Autodesk Inventor part; units mm, degrees
ref_plane "Work Plane1" through (-5, -10, -100) normal (0, 0, -1) x (0, 1, 0)
ref_plane "YZ Plane" through (0, 0, 0) normal (1, 0, 0) x (0, 1, 0)
ref_plane "XZ Plane" through (0, 0, 0) normal (0, 1, 0) x (-1, 0, 0)
sketch "Sketch1" plane through (0, 0, 0) normal (0, 0, 1) x (1, 0, 0)
  line L0 (-5, 10) -> (-5, -10)
  line L1 (-5, -10) -> (5, -10)
  line L2 (5, -10) -> (5, -4)
  line L3 (5, -4) -> (-1, -6.1838)
  line L4 (-1, -6.1838) -> (-1, 6.1838)
  line L5 (-1, 6.1838) -> (5, 4)
  line L6 (5, 4) -> (5, 10)
  line L7 (5, 10) -> (-5, 10)
  line L8 (-1, -10) -> (9, -10)
  line L9 (9, -10) -> (9, 10)
  line L10 (9, 10) -> (-1, 10)
  line L11 (-1, 10) -> (-1, -10)
  point P0 (0, 0)
  dimension "d0" = 10
ref_plane "Work Plane1" through (-5, -10, -100) normal (0, 0, -1) x (0, 1, 0)
extrude "Extrusion1" add sketch "Sketch1" against normal up to surface (100 mm away) contours L10 L9 L8 L2 L3 L4 L5 L6
sketch "Sketch2" plane through (0, 0, 0) normal (0, 0, 1) x (1, 0, 0)
  line L0 (9, 10) -> (5, 10)
  line L1 (5, 10) -> (5, 4)
  line L2 (5, 4) -> (-1, 6.1838)
  line L3 (-1, 6.1838) -> (-1, -6.1838)
  line L4 (-1, -6.1838) -> (5, -4)
  line L5 (5, -4) -> (5, -10)
  line L6 (5, -10) -> (9, -10)
  line L7 (9, -10) -> (9, 10)
  line L8 (5, -10) -> (9, -10)
  line L9 (9, -10) -> (-5, -10)
  line L10 (-5, -10) -> (-5, 10)
  line L11 (-5, 10) -> (9, 10)
  line L12 (9, 10) -> (9, -10)
  point P0 (0, 0)
  dimension "d3" = 14
  dimension "d4" = 20
extrude "Extrusion2" add sketch "Sketch2" along normal blind 3
sketch "Sketch3" plane through (9, -10, -100) normal (1, 0, 0) x (0, 0, -1)
  line L0 (-100, 16.1838) -> (-100, 3.8162)
  circle A0 centre (-94, 10) radius 1.5
  line L1 (0, 0) -> (-103, 0)
  circle A1 centre (-86, 10) radius 1.5
  circle A2 centre (-78, 10) radius 1.5
  circle A3 centre (-70, 10) radius 1.5
  circle A4 centre (-62, 10) radius 1.5
  circle A5 centre (-54, 10) radius 1.5
  circle A6 centre (-46, 10) radius 1.5
  circle A7 centre (-38, 10) radius 1.5
  circle A8 centre (-30, 10) radius 1.5
  circle A9 centre (-22, 10) radius 1.5
  circle A10 centre (-14, 10) radius 1.5
  circle A11 centre (-6, 10) radius 1.5
  point P0 (-100, 10)
  dimension "d7" = 3
  dimension "d8" = 6
  dimension "d11" = 8
extrude "Extrusion3" cut sketch "Sketch3" against normal through all
sketch "Sketch4" plane through (0, 0, 3) normal (0, 0, 1) x (1, 0, 0)
  line L0 (-5, 10) -> (-5, -10)
  line L1 (-5, 10) -> (9, -10)
  line L2 (9, 10) -> (5, 10)
  line L3 (9, -10) -> (9, 10)
  line L4 (-5, -10) -> (5, -10)
  line L5 (9, 10) -> (-5, -10)
  line L6 (-0.75, -2.75) -> (4.75, -2.75)
  line L7 (4.75, -2.75) -> (4.75, 2.75)
  line L8 (4.75, 2.75) -> (-0.75, 2.75)
  line L9 (-0.75, 2.75) -> (-0.75, -2.75)
  line L10 (-0.75, -2.75) -> (4.75, 2.75) construction
  line L11 (4.75, -2.75) -> (-0.75, 2.75) construction
  point P0 (0, 0)
  point P1 (2, 0)
  dimension "d18" = 5.5
  dimension "d19" = 5.5
extrude "Extrusion4" add sketch "Sketch4" along normal blind 7 contours L8 L5 L1 | L1 L5 L6 L9 L8 | L5 L1 L6 | L5 L8 L7 L6 L1
properties part number "prismatic link outer"
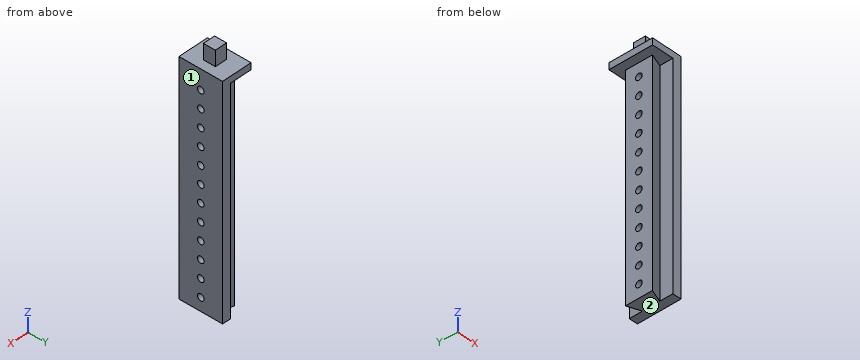
For this review, take the finished solid that the model builds, in its own axes (mm). Face numbers are marked on the shaded views. Round coordinates to 2 decimals unless told otherwise and drop trailing zeros. Loops run counter-clockwise (first coordinate to the right, second up) from the corner with the lowest first, then second, coordinate; pieces in that order, holes last. Notation, with made-up numbers: (-24, 69) - (-2, 69) arc R37 ccw to (-2, 106) - close; hole circle Ø5 at (-36, -7). An arc over 180 degrees is marked (long way). Put each result on its own line as item: value. Start each with the question number.
1. Consider section C-C on x = 3.5. State how many separate pieces and enclosed holes the cut face has, plus the area to 3 significant figures.
2. For probe 1 along Z at (x, y) = (8.5, 5.5); probe 2 along Y at (x, z) = (0.75, 3.5); probe 3 along Y at (x, z) = (5.5, -38), list the stretches that pass through material, from the lowest coordinate up. Write a range as [from, to].
3. Consider section D-D on x = -2.5. State the section outline as (y, z) points.
4. Consider section A-A on z = -6. State the section outline as (x, y) points, plus the area to 3 significant figures.
5. Mouldability with a two-part tool opening along Z and no side actions: class the marked faces 1 and 2 as +Z half, -Z half, draft (parallel to the pull), parting line (faces both ways), or undercut.
6. Consider section B-B on z = -42. State the section outline as (x, y) points.
7. Insertion check: P1, Ø1.6, axis at x = 2.5, z = 7.5, coming from the +Y side; P2, Ø8, axis at y = 5, z = -81, coming from the -X side; P3, Ø3, axis at x = 3, z = 7, coming from the -Y side. Each pin has a flat end and moves straight along its axis. Give the tip position at first contact, or say it passes through.
Result sheet:
1. separate pieces: 1
1. enclosed holes: 12
1. area: 923 mm^2
2. probe 1: [-100, 3]
2. probe 2: [-2.75, 2.75]
2. probe 3: [-10, -1.5], [1.5, 10]
3. outline: (-10, 0) - (10, 0) - (10, 3) - (-10, 3) - close
4. outline: (-1, -6.18) - (5, -4) - (5, -10) - (9, -10) - (9, -1.5) - (-1, -1.5) - close; (-1, 1.5) - (9, 1.5) - (9, 10) - (5, 10) - (5, 4) - (-1, 6.18) - close
4. area: 111 mm^2
5. face 1: draft
5. face 2: -Z half
6. outline: (-1, -6.18) - (5, -4) - (5, -10) - (9, -10) - (9, 10) - (5, 10) - (5, 4) - (-1, 6.18) - close
7. P1: y = 2.75
7. P2: x = -1
7. P3: y = -2.75
